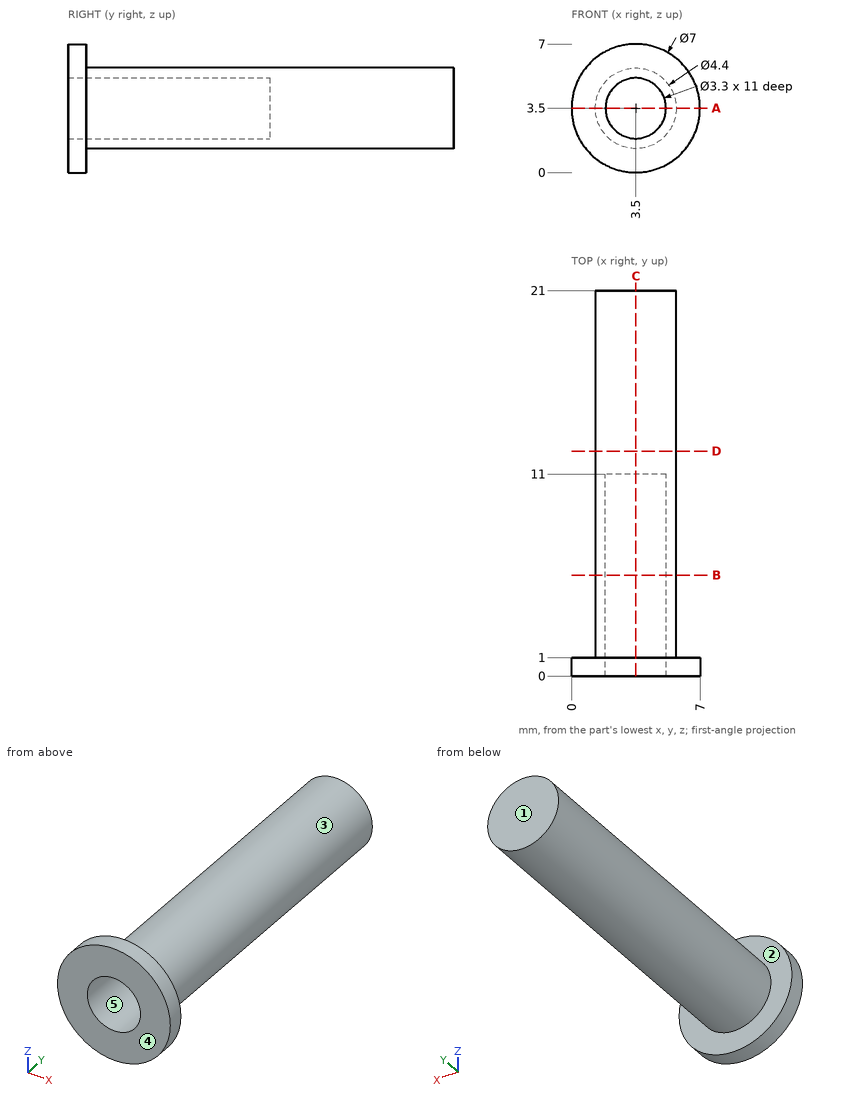
The figure shows three views and two pictorial views of one solid part (mm, origin at its lowest corner). Answer the questions. A direction names the side the tool comes from. Give positions to 0.01 mm unless a question says otherwise; leave off trailing zeros. Order: outer loops, then holes, each group sorted by start corner. A loop starts at its lowest first (then second) coordinate and runs counter-clockwise, first axis right, second up. Notation, with made-up numbers: (45, 35) -> (70, 35) arc R14 ccw to (70, 54) -> close; hole circle Ø5 at (36, 72.25). An arc over 180 degrees is marked (long way). Answer as a JSON object with one key per item and string values. Group by question number.
Item 1: The part is cut by section A-A on z = 3.5. Write down the section's boundary in (x, y), and give its area (3 significant figures).
Item 2: The part is cut by section D-D on y = 12.25. Write down the section's boundary in (x, z), and give its area (3 significant figures).
Item 3: Consider L1, parallel to Z at x = 3.5, y = 7.75; L2, parallel to Y at x = 0.5, z = 1.75; L3, parallel to X at y = 10.5, z = 2.75. Determine where each line is inside the solid, lowest interval first. Write a range as from..to.
Item 4: The part is cut by section B-B on y = 5.5. Write down the section's boundary in (x, z), and give its area (3 significant figures).
Item 5: Determine the mould class of the marked faces 3, 4 and 5 for opening direction Z: pulls with the +Z half, pulls with the -Z half, needs draft (parallel to the pull), parting line crosses it, or undercut.
Item 6: The part is cut by section C-C on x = 3.5. Write down the section's boundary in (y, z), and give its area (3 significant figures).
Item 7: A tool of negligible diameter and unlimited length cuts with its end or side. For the marked faces 1 and 2, from which of +Z, -Z, +X, -X, +Y, -Y can it reach the whole face along a straight path? Write none if from no direction.
Item 8: Flat-ended cylindrical pins translate along their axes: pin 1 (3 mm diameter, centred on x = 5, y = 11.5, fed in from -Z); pin 2 (4 mm diameter, centred on x = 2, z = 5.5, fed in from +Y); pin 3 (4 mm diameter, centred on y = 16, z = 3.5, fed in from +X); pin 4 (2 mm diameter, centred on y = 12, z = 6, fed in from +X). Find the tip coordinate at first contact, or state that the pin passes through.
Result set:
{
 "1": {"outline": "(0, 0) -> (1.85, 0) -> (1.85, 11) -> (5.15, 11) -> (5.15, 0) -> (7, 0) -> (7, 1) -> (5.7, 1) -> (5.7, 21) -> (1.3, 21) -> (1.3, 1) -> (0, 1) -> close", "area": "58.7 mm²"},
 "2": {"outline": "circle Ø4.4 at (3.5, 3.5)", "area": "15.2 mm²"},
 "3": {"L1": "1.3..1.85, 5.15..5.7", "L2": "0..1", "L3": "1.43..2.03, 4.97..5.57"},
 "4": {"outline": "circle Ø4.4 at (3.5, 3.5); hole circle Ø3.3 at (3.5, 3.5)", "area": "6.65 mm²"},
 "5": {"face 3": "parting line crosses it", "face 4": "needs draft", "face 5": "undercut"},
 "6": {"outline": "(0, 0) -> (1, 0) -> (1, 1.3) -> (21, 1.3) -> (21, 5.7) -> (1, 5.7) -> (1, 7) -> (0, 7) -> (0, 5.15) -> (11, 5.15) -> (11, 1.85) -> (0, 1.85) -> close", "area": "58.7 mm²"},
 "7": {"face 1": "+Z, -Z, +X, -X, +Y", "face 2": "+Y"},
 "8": {"pin 1": "z = 1.3", "pin 2": "y = 21", "pin 3": "x = 5.7", "pin 4": "x = 5.11"}
}
